```python
from build123d import *

# Parameters (mm, degrees)
F0_R     = 1
F0_W     = 10
F0_H     = 3.5
F0_W_2   = 6.1
F0_H_2   = 6.1
F0_R_2   = 1.5
F0_R_3   = 1.75
F1_DEPTH = 1.5
F2_DEPTH = 4.3
F3_DEPTH = 7.3
F4_DEPTH = 5
F5_DEPTH = 3.3


with BuildPart() as f1:
    # F0 (on Top) → F1 (new body)
    with BuildSketch(Plane.XY):
        Polygon((16.5, 24.617638), (-16.5, 24.617638), (-16.5, -17.682362), (0, -17.682362), (16.5, -17.682362), align=None)
        with Locations((-13.9, -11.682362)):
            Circle(F0_R, mode=Mode.SUBTRACT)
        with BuildLine():
            ThreePointArc((10.2, -7.482362), (7.212489, -14.694851), (0, -17.682362))
            ThreePointArc((0, -17.682362), (-7.212489, -0.269872), (10.2, -7.482362))
        make_face(mode=Mode.SUBTRACT)
        with Locations((13.9, -11.682362)):
            Circle(F0_R, mode=Mode.SUBTRACT)
        with Locations((-0.111425, 6.467638)):
            Rectangle(F0_W, F0_H, mode=Mode.SUBTRACT)
        with Locations((-13.9, 22.517638)):
            Circle(F0_R, mode=Mode.SUBTRACT)
        with Locations((0, 12.367638)):
            Rectangle(F0_W_2, F0_H_2, mode=Mode.SUBTRACT)
        with Locations((0, 19.867638)):
            Circle(F0_R_2, mode=Mode.SUBTRACT)
        with Locations((13.9, 22.517638)):
            Circle(F0_R, mode=Mode.SUBTRACT)
        with BuildLine():
            ThreePointArc((10.2, -7.482362), (-7.212489, -0.269872), (0, -17.682362))
            ThreePointArc((0, -17.682362), (7.212489, -14.694851), (10.2, -7.482362))
        make_face()
        with Locations((0, 19.867638)):
            Circle(F0_R_2)
        with Locations((0, 12.367638)):
            Rectangle(F0_W_2, F0_H_2)
        with Locations((0, 12.367638)):
            Circle(F0_R_3, mode=Mode.SUBTRACT)
        with Locations((0, 12.367638)):
            Circle(F0_R_3)
        with Locations((-0.111425, 6.467638)):
            Rectangle(F0_W, F0_H)
    extrude(amount=F1_DEPTH)

    # F0 (on Top) → F2 (join)
    with BuildSketch(Plane.XY):
        with BuildLine():
            ThreePointArc((10.2, -7.482362), (-7.212489, -0.269872), (0, -17.682362))
            ThreePointArc((0, -17.682362), (7.212489, -14.694851), (10.2, -7.482362))
        make_face()
    extrude(amount=-F2_DEPTH)

    # F0 (on Top) → F3 (join)
    with BuildSketch(Plane.XY):
        with Locations((0, 19.867638)):
            Circle(F0_R_2)
        with Locations((0, 12.367638)):
            Circle(F0_R_3)
    extrude(amount=F3_DEPTH)

    # F0 (on Top) → F4 (join)
    with BuildSketch(Plane.XY):
        with Locations((0, 12.367638)):
            Rectangle(F0_W_2, F0_H_2)
        with Locations((0, 12.367638)):
            Circle(F0_R_3, mode=Mode.SUBTRACT)
    extrude(amount=F4_DEPTH)

    # F0 (on Top) → F5 (join)
    with BuildSketch(Plane.XY):
        with Locations((-0.111425, 6.467638)):
            Rectangle(F0_W, F0_H)
    extrude(amount=-F5_DEPTH)


solid = f1.part
```
Build history of the part. All positions in model axes, mm. A direction names the side the tool comes from. Round coordinates to 2 decimals unless told otherwise and drop trailing zeros. Loops run counter-clockwise (first coordinate to the right, second up) from the corner with the lowest first, then second, coordinate; pieces in that order, holes last.
Item 1: Drill centre lines: line 1 along Y through (x, z) = (-13.9, 0.85); line 2 along Z through (x, y) = (-10.5, -6.5); line 3 along Z through (x, y) = (1.5, -9). Where is each one in solid material? Low to high.
Item 2: Which spindle directions (+Z, -Z, +X, -X, +Y, -Y) get a long thin tool onto all of the face, cutting with end or side? Do faces 4 (the face through (-3.05, 12, 3)), 5 (the face through (-5.111, 6, -2)), 6 (the face through (0, 9.318, 3)), 7 (the face through (0, 8.218, -2)). Say none if no direction does.
Item 3: Saw through at A-A (z = -2). List the corners of the cut face in (x, y).
Item 4: Pin check, flat tips, straight feed: P1, Ø3, axis at x = 0, y = 7, coming from the -Z side; P2, Ø1, axis at y = 11, z = 3.5, coming from the -X side; P3, Ø1, axis at y = 7, z = -1, coming from the -X side; P4, Ø10, axis at x = 0, y = 7, coming from the -Z side. Stop position of each tip, or through.
Item 5: Saw through at C-C (y = -14.5). List the corners of the cut face in (x, z).
Item 6: Two-plate mould, pull along X, no slides. Class faces 1 (the face through (0, 20, 7.3)), 2 (the face through (13.106, 21.909, 0.74)), 3 (the face through (-0.228, 14.103, 6.134)): released by +X, released by -X, zero draft, split by the parting line, or undercut.
Item 7: Saw through at B-B (x = -13.9). List the corners of the cut face in (y, z), then the cut area to 4 significant figures.
Item 8: Saw through at D-D (x = -9.5). List the corners of the cut face in (y, z).
Worked answers:
1. line 1: y = -17.68 to -12.68, -10.68 to 21.52, 23.52 to 24.62
1. line 2: z = 0 to 1.5
1. line 3: z = -4.3 to 1.5
2. face 4: +Z, -X, +Y, -Y
2. face 5: -Z, -X, +Y
2. face 6: +Z, +X, -X, -Y
2. face 7: -Z, +X, -X, +Y
3. outline: circle Ø20.4 at (0, -7.48); (-5.11, 4.72) - (4.89, 4.72) - (4.89, 8.22) - (-5.11, 8.22) - close
4. P1: stops at z = -3.3
4. P2: stops at x = -3.05
4. P3: stops at x = -5.11
4. P4: stops at z = -4.3
5. outline: (-16.5, 0) - (-7.4, 0) - (-7.4, -4.3) - (7.4, -4.3) - (7.4, 0) - (16.5, 0) - (16.5, 1.5) - (-16.5, 1.5) - close
6. face 1: zero draft
6. face 2: undercut
6. face 3: split by the parting line
7. outline: (-17.68, 0) - (-12.68, 0) - (-12.68, 1.5) - (-17.68, 1.5) - close; (-10.68, 0) - (21.52, 0) - (21.52, 1.5) - (-10.68, 1.5) - close; (23.52, 0) - (24.62, 0) - (24.62, 1.5) - (23.52, 1.5) - close
7. area: 57.45 mm2
8. outline: (-17.68, 0) - (-11.2, 0) - (-11.2, -4.3) - (-3.77, -4.3) - (-3.77, 0) - (24.62, 0) - (24.62, 1.5) - (-17.68, 1.5) - close
